```python
from build123d import *

# Parameters (mm, degrees)
SKETCH1_W          = 10
SKETCH1_H          = 10
EXTRUDE1_DEPTH     = 600
SKETCH2_R          = 2
CUT_EXTRUDE1_DEPTH = 20
CUT_EXTRUDE2_START = -20
SKETCH3_R          = 2
CUT_EXTRUDE2_DEPTH = 20
SKETCH4_R          = 1.5
CUT_EXTRUDE3_DEPTH = 601.166643525
LPATTERN1_COUNT    = 10
LPATTERN1_PITCH    = 60


with BuildPart() as part:
    # Sketch1 → Extrude1 (new body)
    with BuildSketch(Plane.XY):
        with Locations((5, 5)):
            Rectangle(SKETCH1_W, SKETCH1_H)
    extrude(amount=EXTRUDE1_DEPTH)

    # Sketch2 → Cut-Extrude1 (cut)
    with BuildSketch(Plane.XY.offset(600)):
        with Locations((5, 5)):
            Circle(SKETCH2_R)
    extrude(amount=-CUT_EXTRUDE1_DEPTH, mode=Mode.SUBTRACT)

    # Sketch3 → Cut-Extrude2 (cut)
    with BuildSketch(Plane(origin=(0, 0, 0), x_dir=(-1, 0, 0), z_dir=(0, 0, -1)).offset(CUT_EXTRUDE2_START)):
        with Locations(Location((-5, 5, 0), (0, 0, 180))):
            Circle(SKETCH3_R)
    extrude(amount=CUT_EXTRUDE2_DEPTH, mode=Mode.SUBTRACT)

    # Sketch4 → Cut-Extrude3 (cut, through all)
    with BuildSketch(Plane(origin=(0, 10, 0), x_dir=(-1, 0, 0), z_dir=(0, 1, 0))):
        with Locations(Location((-5, 30, 0), (0, 0, 90))):
            Circle(SKETCH4_R)
    cut_extrude3 = extrude(amount=-CUT_EXTRUDE3_DEPTH, mode=Mode.SUBTRACT)

    # LPattern1: Cut-Extrude3 ×10
    with Locations(*[(0, 0, i * LPATTERN1_PITCH) for i in range(1, LPATTERN1_COUNT)]):
        add(cut_extrude3, mode=Mode.SUBTRACT)


solid = part.part
```
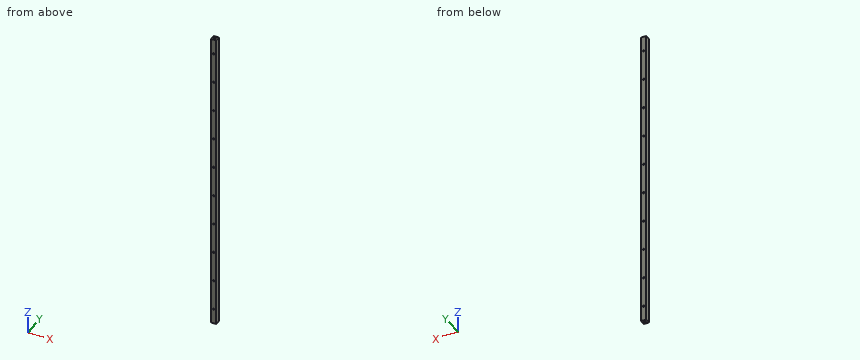
Can you work these out from the model? Positions are in its coordinate system, mm. Coordinates: 2 decimals unless noted, no trailing zeros. Return JSON: item names as keys, results as strings.
Q1. If we section it at A-A (y = 5): Count the separate pieces of the cut face and the enclosed holes in it, then the cut area to 3 significant figures.
Computed values:
{"separate pieces": "1", "enclosed holes": "10", "area": "5,770 mm2"}
Q2. Please list where these lines run through material, in increasing order: L1, parallel to X at y = 5, z = 9.5; L2, parallel to X at y = 7, z = 210. Write a range as from..to.
Computed values:
{"L1": "x = 0..3, 7..10", "L2": "x = 0..3.5, 6.5..10"}
Q3. I'm going to push flat-ended pins straight in: pin 1 Ø2 at (x, z) = (8, 534) entering from -Y; pin 2 Ø2.5 at (x, z) = (5, 330) entering from -Y; pin 3 Ø3 at (x, y) = (5, 5) entering from -Z; pin 4 Ø2 at (x, y) = (5.5, 5) entering from +Z. Where does each tip first touch, or does it pass through?
Computed values:
{"pin 1": "stops at y = 0", "pin 2": "passes through", "pin 3": "stops at z = 20", "pin 4": "stops at z = 580"}
